The listing builds one solid part. Answer for the finished solid, in the listing's coordinates (mm). A direction names the side the tool comes from. Give positions to 0.01 mm unless a question says otherwise; leave off trailing zeros. Loops run counter-clockwise (first coordinate to the right, second up) from the corner with the lowest first, then second, coordinate; pieces in that order, holes last. Notation, with made-up numbers: (10.25, 31) - (45.25, 31) arc R19 cw to (45.25, 67) - close; hole circle Ø11 at (-1.75, 53.25). An arc over 180 degrees is marked (long way). Answer as CSV lines item,"result". Start each with the question number.
1) A cutting plane is placed at B-B (z = 0). Determine the outline of the cut face in (x, y).
2) A cutting plane is placed at C-C (y = 1.5). Determine the outline of the cut face in (x, z).
3) A cutting plane is placed at A-A (x = 0). Determine the outline of the cut face in (y, z), and give its area (3 significant figures).
4) For faces 1 (the face through (3.434, 6.479, 1.081)), 2 (the face through (-11, 1, -2)), 3 (the face through (12, 1, 2)), 4 (the face through (-12, 3, 0)), 5 (the face through (-12, 1, 2)), determine the directions among +Z, -Z, +X, -X, +Y, -Y from which every point of the face is accessible in a straight line to the end or side of a thin tool.
5) A cutting plane is placed at D-D (y = 3.5). Determine the outline of the cut face in (x, z).
6) Find the intervals of material crossed by line 1 along Y through (x, z) = (-5.25, -2.75); line 2 along X through (y, z) = (4, -2); line 3 along Z through (x, y) = (-2, 0.5), in increasing order.
7) Flat-ended cylindrical pins translate along their axes: pin 1 (0.9 mm diameter, centred on x = 11.5, z = 1, fed in from +Y); pin 2 (5 mm diameter, centred on x = 4, z = 0, fed in from +Y); pin 3 (0.7 mm diameter, centred on x = -9.5, y = 1.5, fed in from +Z); pin 4 (2.5 mm diameter, centred on x = 11, y = 2, fed in from +Z). Find the tip coordinate at first contact, or state that the pin passes through.
Autodesk Inventor part; units mm, degrees
ref_plane "YZ Plane" through (0, 0, 0) normal (1, 0, 0) x (0, 1, 0)
ref_plane "XZ Plane" through (0, 0, 0) normal (0, 1, 0) x (-1, 0, 0)
ref_plane "XY Plane" through (0, 0, 0) normal (0, 0, 1) x (1, 0, 0)
sketch "Sketch1" plane through (0, 0, 0) normal (0, 1, 0) x (-1, 0, 0)
  circle A0 centre (0, 0) radius 10
  dimension "d0" = 20
extrude "Extrusion1" add sketch "Sketch1" along normal blind 5
sketch "Sketch2" plane through (0, 5, 0) normal (0, 1, 0) x (1, 0, 0)
  line L0 (-14, 0) -> (14, 0)
  line L1 (0, 14) -> (0, -14)
  circle A0 centre (0, 0) radius 3.6
  dimension "d3" = 7.2
extrude "Extrusion2" add sketch "Sketch2" along normal blind 3
sketch "Sketch3" plane through (0, 0, 0) normal (0, -1, 0) x (1, 0, 0)
  line L0 (10, -3.5) -> (-10, -3.5)
  line L1 (-10, -3.5) -> (-10, 3.5)
  line L2 (-10, 3.5) -> (10, 3.5)
  line L3 (10, 3.5) -> (10, -3.5)
  circle A0 centre (0, 0) radius 10
  circle A1 centre (0, 0) radius 10
  line L4 (-14, 0) -> (14, 0)
  line L5 (0, -14) -> (0, 14)
  line L6 (10, -2) -> (13, -2)
  line L7 (13, -2) -> (13, 2)
  line L8 (13, 2) -> (10, 2)
  line L9 (-10, -2) -> (-13, -2)
  line L10 (-13, -2) -> (-13, 2)
  line L11 (-13, 2) -> (-10, 2)
  dimension "d6" = 7
  dimension "d7" = 4
  dimension "d8" = 3
  dimension "d9" = 4
  dimension "d10" = 3
extrude "Extrusion3" add sketch "Sketch3" against normal up to surface (5 mm away) contours L0 A0 L3 | L0 L5 L4 A0 | L0 A0 L4 L5 | A0 L2 L3 | L4 L5 L2 A0 | L0 L1 A0 | L4 A0 L2 L5 | L1 L2 A0
extrude "Extrusion4" add sketch "Sketch3" against normal blind 3 contours L3 L4 L7 L6 | L3 L8 L7 L4 | L4 L10 L11 L1 | L1 L9 L10 L4
sketch "Sketch4" plane through (0, 0, 0) normal (0, -1, 0) x (1, 0, 0)
  arc A0 (9.3675, 3.5) -> (-9.3675, 3.5) centre (0, 0) ccw
  line L0 (-9.3675, 3.5) -> (-10, 3.5)
  line L1 (-10, 3.5) -> (-10, 2)
  line L2 (-10, 2) -> (-13, 2)
  line L3 (-13, 2) -> (-13, -2)
  line L4 (-13, -2) -> (-10, -2)
  line L5 (-10, -2) -> (-10, -3.5)
  line L6 (-10, -3.5) -> (-9.3675, -3.5)
  arc A1 (-9.3675, -3.5) -> (9.3675, -3.5) centre (0, 0) ccw
  line L7 (9.3675, -3.5) -> (10, -3.5)
  line L8 (10, -3.5) -> (10, -2)
  line L9 (10, -2) -> (13, -2)
  line L10 (13, -2) -> (13, 2)
  line L11 (13, 2) -> (10, 2)
  line L12 (10, 2) -> (10, 3.5)
  line L13 (10, 3.5) -> (9.3675, 3.5)
  line L14 (0, -31.9933) -> (0, 47.9155)
  line L15 (-29.75, 0) -> (29.75, 0)
  arc A2 (9.3675, 3.5) -> (-9.3675, 3.5) centre (0, 0) ccw
  circle A3 centre (0, 15.25) radius 21.25
  line L16 (15.0443, -6) -> (-18.096, -6) construction
  line L17 (10.2288, -3.7354) -> (10.2288, -20.5777)
  line L18 (10.2288, -20.5777) -> (-9.5456, -20.5777)
  line L19 (-9.5456, -20.5777) -> (-9.5456, -3.7354)
  line L20 (-9.5456, -3.7354) -> (-9.2762, -3.7354)
  line L21 (9.5456, -3.7354) -> (10.2288, -3.7354)
  dimension "d16" = 6
extrude "Extrusion5" cut sketch "Sketch4" against normal through all contours A3 A1 L14 | L14 A1 A3 | L14 L18 L19 A3 A1 | A1 A3 L21 L17 L18 L14
properties part number "turntable"
Ans:
1,outline,"(-13, 0) - (13, 0) - (13, 3) - (10, 3) - (10, 5) - (3.6, 5) - (3.6, 8) - (-3.6, 8) - (-3.6, 5) - (-10, 5) - (-10, 3) - (-13, 3) - close"
2,outline,"(-13, -2) - (-10, -2) - (-10, -3.5) - (-9.37, -3.5) arc R10 ccw to (-9.21, -3.9) arc R21.25 ccw to (9.21, -3.9) arc R10 ccw to (9.37, -3.5) - (10, -3.5) - (10, -2) - (13, -2) - (13, 2) - (10, 2) - (10, 3.5) - (9.37, 3.5) arc R10 ccw to (-9.37, 3.5) - (-10, 3.5) - (-10, 2) - (-13, 2) - close"
3,outline,"(0, -6) - (5, -6) - (5, -3.6) - (8, -3.6) - (8, 3.6) - (5, 3.6) - (5, 10) - (0, 10) - close"
3,area,"102 mm2"
4,face 1,"+Y"
4,face 2,"-Z, -X, +Y, -Y"
4,face 3,"+Z, +X, +Y, -Y"
4,face 4,"+Z, -Z, -X, +Y"
4,face 5,"+Z, -X, +Y, -Y"
5,outline,"(-10, -3.5) - (-9.37, -3.5) arc R10 ccw to (-9.21, -3.9) arc R21.25 ccw to (9.21, -3.9) arc R10 ccw to (9.37, -3.5) - (10, -3.5) - (10, 3.5) - (9.37, 3.5) arc R10 ccw to (-9.37, 3.5) - (-10, 3.5) - close"
6,line 1,"0 to 5"
6,line 2,"-10 to 10"
6,line 3,"-5.91 to 9.8"
7,pin 1,"y = 3"
7,pin 2,"y = 8"
7,pin 3,"z = 4.03"
7,pin 4,"z = 3.5"
